Autodesk Inventor part; units mm, degrees
ref_plane "YZ Plane" through (0, 0, 0) normal (1, 0, 0) x (0, 1, 0)
ref_plane "XZ Plane" through (0, 0, 0) normal (0, 1, 0) x (-1, 0, 0)
ref_plane "XY Plane" through (0, 0, 0) normal (0, 0, 1) x (1, 0, 0)
sketch "Sketch1" plane through (0, 0, 0) normal (0, 0, 1) x (1, 0, 0)
  line L0 (0, 0) -> (-85, 0)
  line L1 (-85, 0) -> (-85, 85)
  line L2 (-85, 85) -> (0, 85)
  line L3 (0, 85) -> (0, 0)
  dimension "d0" = 85
  dimension "d1" = 85
extrude "Extrusion1" add sketch "Sketch1" along normal blind 175
fillet "Fillet2" radius 3.175 8 edges at (-85, 42.5, 175) (0, 42.5, 175) (-42.5, 0, 175) (-85, 0, 87.5) (0, 0, 87.5) (0, 42.5, 0) (-42.5, 0, 0) (-85, 42.5, 0)
shell "Shell1" thickness 2.54 removed faces 1 at (-28.3333, 85, 59.3917)
sketch "Sketch2" plane through (-81.825, 85, 0) normal (0, 1, 0) x (1, 0, 0)
  line L0 (-2.54, -175) -> (81.19, -175)
  line L1 (81.19, -175) -> (81.19, -0.635)
  line L2 (81.19, -0.635) -> (-2.54, -0.635)
  line L3 (-2.54, -0.635) -> (-2.54, -175)
  point P0 (81.825, 0)
  point P1 (0, -172.46)
  point P2 (78.65, -3.175)
extrude "Extrusion2" add sketch "Sketch2" along normal blind 2.54
fillet "Fillet3" radius 3.175 4 edges at (-84.365, 86.27, 175) (-0.635, 86.27, 175) (-0.635, 86.27, 0.635) (-84.365, 86.27, 0.635)
properties part number "AC_power_box" material "Iron, Cast"
Part model, mm, in its own coordinate system. A direction names the side the tool comes from. Coordinates: 2 decimals unless noted, no trailing zeros. Write each loop counter-clockwise with the first axis right and the second up, starting at its lowest first coordinate (ties: lowest second). Pieces come first, ordered by that corner, then holes.
Item 1: Slice it at C-C (z = 25.5). Write the cut outline in (x, y) (3 decimals).
Item 2: Which spindle directions (+Z, -Z, +X, -X, +Y, -Y) get a long thin tool onto all of the face, cutting with end or side? Do faces 1 (the face through (-2.54, 45, 86)), 2 (the face through (-43, 87.54, 87)). Say none if no direction does.
Item 3: Probe line 1 (Z direction, x = -43.5, y = 56.5); line 2 (Y direction, x = -69, z = 126); line 3 (X direction, y = 77, z = 117.5). List the from-to ranges inside material, lowest first.
Item 4: Mould opens along Z. For faces 3 (the face through (-42, 0, 86)), 4 (the face through (-43, 46, 175)), 5 (the face through (-43, 45, 0)), 6 (the face through (-43, 85, 86)) say: released by +Z, released by -Z, zero draft, split by the parting line, or undercut.
Item 5: Slice it at A-A (x = -64). Write the cut outline in (y, z) (3 decimals).
Item 6: Pin check, flat tips, straight feed: pin 1 (0.8 mm diameter, centred on y = 86, z = 68.5, fed in from +X) (3 decimals); pin 2 (2 mm diameter, centred on x = -61, y = 86.5, fed in from -Z) (3 decimals); pin 3 (1.3 mm diameter, centred on y = 86, z = 61, fed in from -X) (3 decimals). Stop position of each tip, or through.
Item 7: Slice it at B-B (y = 71). Write the cut outline in (x, z) (3 decimals), and give its area (3 significant figures).
Results found:
1. outline: (-85, 3.175) arc R3.175 ccw to (-81.825, 0) - (-3.175, 0) arc R3.175 ccw to (0, 3.175) - (0, 85) - (-0.635, 85) - (-0.635, 87.54) - (-84.365, 87.54) - (-84.365, 85) - (-85, 85) - close; hole (-82.46, 3.175) arc R0.635 ccw to (-81.825, 2.54) - (-3.175, 2.54) arc R0.635 ccw to (-2.54, 3.175) - (-2.54, 85) - (-82.46, 85) - close
2. face 1: none
2. face 2: +Z, -Z, +X, -X, +Y
3. line 1: z = 0 to 2.54, 172.46 to 175
3. line 2: y = 0 to 2.54, 85 to 87.54
3. line 3: x = -85 to -82.46, -2.54 to 0
4. face 3: zero draft
4. face 4: released by +Z
4. face 5: released by -Z
4. face 6: undercut
5. outline: (0, 3.175) arc R3.175 ccw to (3.175, 0) - (85, 0) - (85, 0.635) - (87.54, 0.635) - (87.54, 175) - (3.175, 175) arc R3.175 ccw to (0, 171.825) - close; hole (2.54, 3.175) arc R0.635 ccw to (3.175, 2.54) - (85, 2.54) - (85, 172.46) - (3.175, 172.46) arc R0.635 ccw to (2.54, 171.825) - close
6. pin 1: stops at x = -0.635
6. pin 2: stops at z = 0.635
6. pin 3: stops at x = -84.365
7. outline: (-85, 3.175) arc R3.175 ccw to (-81.825, 0) - (-3.175, 0) arc R3.175 ccw to (0, 3.175) - (0, 171.825) arc R3.175 ccw to (-3.175, 175) - (-81.825, 175) arc R3.175 ccw to (-85, 171.825) - close; hole (-82.46, 3.175) arc R0.635 ccw to (-81.825, 2.54) - (-3.175, 2.54) arc R0.635 ccw to (-2.54, 3.175) - (-2.54, 171.825) arc R0.635 ccw to (-3.175, 172.46) - (-81.825, 172.46) arc R0.635 ccw to (-82.46, 171.825) - close
7. area: 1,290 mm2
